The figure shows three views and two pictorial views of one solid part (mm, origin at its lowest corner). Answer the questions. Coordinates: 2 decimals unless noted, no trailing zeros. Write each loop counter-clockwise with the first axis right and the second up, starting at its lowest first coordinate (ties: lowest second). Pieces come first, ordered by that corner, then holes. Notation, with made-up numbers: M 79,53.25 L 92,53.25 A27 ccw 92,86.25 Z; hole C 77,41.25 d11. An arc over 180 degrees is marked long. Use CSV: the item, a comma, the result in double quotes.
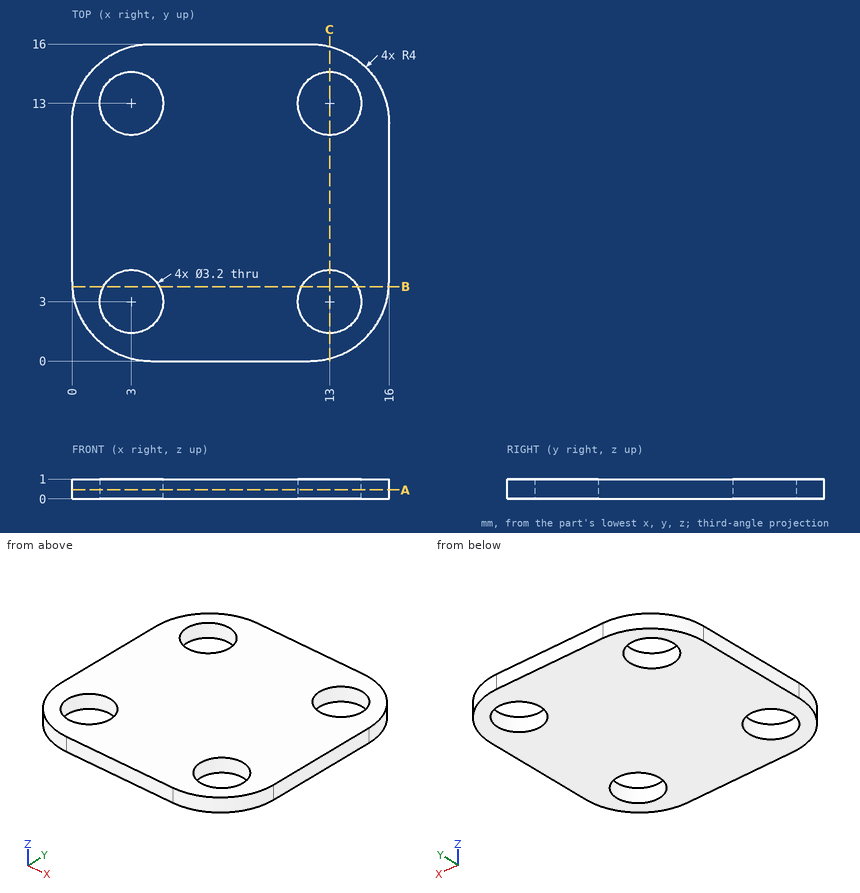
Item 1: The part is cut by section C-C (x = 13). Write down the section's boundary in (y, z), then the cut area to 3 significant figures.
Answer:
outline,"M 0.13,0 L 1.4,0 L 1.4,1 L 0.13,1 Z; M 4.6,0 L 11.4,0 L 11.4,1 L 4.6,1 Z; M 14.6,0 L 15.87,0 L 15.87,1 L 14.6,1 Z"
area,"9.35 mm2"
Item 2: Consider probe 1 along Y at (x, z) = (2, 0.2); probe 2 along X at (y, z) = (1.75, 0.4); probe 3 along X at (y, z) = (13, 0.5). Determine where each line is inside the solid, lowest interval first.
Answer:
probe 1,"y = 0.54 to 1.75, 4.25 to 11.75, 14.25 to 15.46"
probe 2,"x = 0.69 to 2, 4 to 12, 14 to 15.31"
probe 3,"x = 0.13 to 1.4, 4.6 to 11.4, 14.6 to 15.87"
Item 3: The part is cut by section A-A (z = 0.45). Write down the section's boundary in (x, y).
Answer:
outline,"M 0,4 A4 ccw 4,0 L 12,0 A4 ccw 16,4 L 16,12 A4 ccw 12,16 L 4,16 A4 ccw 0,12 Z; hole C 3,3 d3.2; hole C 3,13 d3.2; hole C 13,3 d3.2; hole C 13,13 d3.2"
Item 4: The part is cut by section B-B (y = 3.75). Write down the section's boundary in (x, z).
Answer:
outline,"M 0.01,0 L 1.59,0 L 1.59,1 L 0.01,1 Z; M 4.41,0 L 11.59,0 L 11.59,1 L 4.41,1 Z; M 14.41,0 L 15.99,0 L 15.99,1 L 14.41,1 Z"
Item 5: Given pin 1 (1.9 mm diameter, centred on x = 13, y = 13, fed in from -Z); pin 2 (1 mm diameter, centred on x = 3, y = 11.5, fed in from -Z), each flat-ended and moving along its own axis, determine where each tip first touches the part or whether it passes through.
Answer:
pin 1,"passes through"
pin 2,"stops at z = 0"
